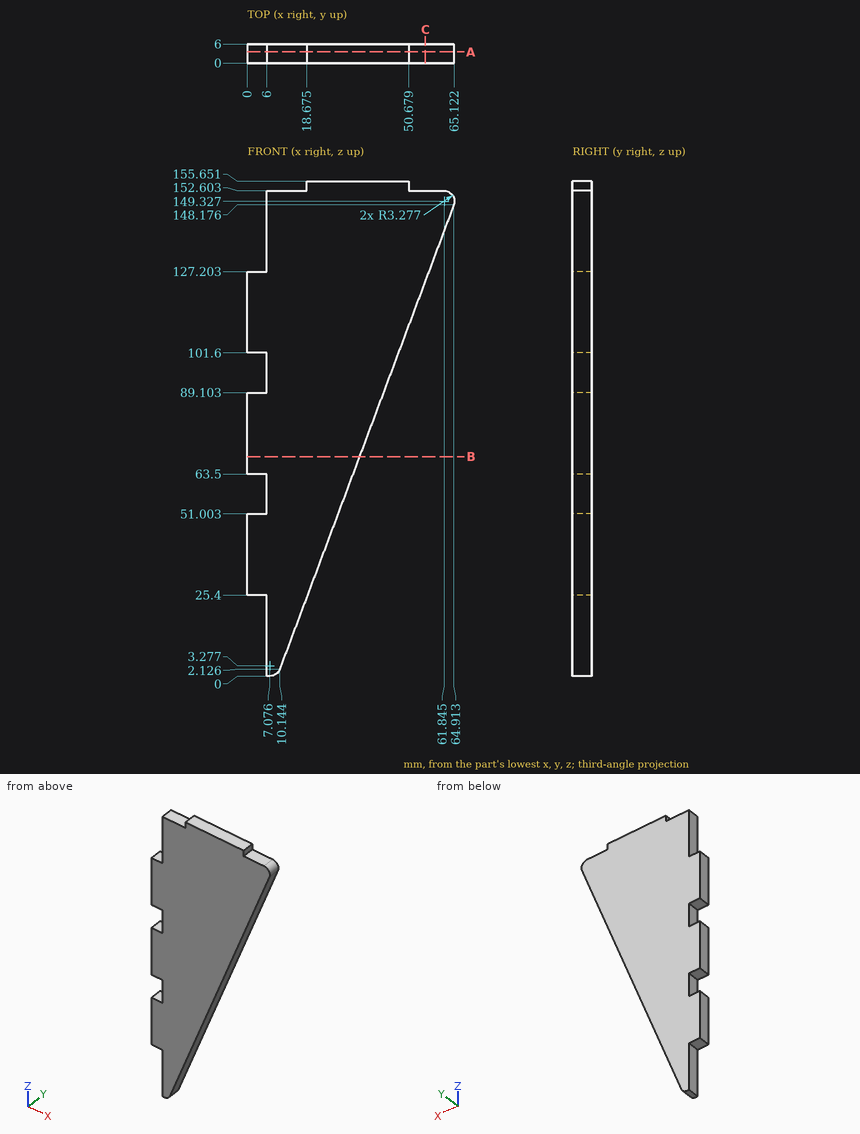
Design review of the part shown in the three views and the two pictorial views. Dimensions are in mm from the part's minimum x, y and z. Round coordinates to 2 decimals unless told otherwise and drop trailing zeros. Order: outer loops, then holes, each group sorted by start corner. A loop starts at its lowest first (then second) coordinate and runs counter-clockwise, first axis right, second up. Notation, with made-up numbers: (64, -7) - (115, -7) arc R23 ccw to (115, 22) - close; hole circle Ø8 at (85.25, -38). An arc over 180 degrees is marked (long way). One line per question, with ' | ' between items.
Item 1: For P1, Ø1.8, axis at x = 3, y = 4.5, coming from the -Z side; P2, Ø1.8, axis at y = 4, z = 58, coming from the -X side; P3, Ø3, axis at x = 2.5, y = 2, coming from the +Z side; P4, Ø3, axis at x = 33, z = 86.5, coming from the -Y side, all flat-tipped, find the tip position at first contact; note any pin that passes through.
Checks:
P1: z = 25.4 | P2: x = 6 | P3: z = 127.2 | P4: y = 0
Item 2: Take a section at C-C, the plane x = 56. Write out the cut boundary in (y, z).
Checks:
outline: (0, 124.41) - (6, 124.41) - (6, 152.6) - (0, 152.6) - close
Item 3: Wall thickness on line 1 (Z direction, x = 4, y = 1.4); line 2 (X direction, y = 5.6, z = 144.5) (1 decimal); line 3 (X direction, y = 1.25, z = 119): over which ranges is each line inside the solid? List them lowest first. Write a range as [from, to].
Checks:
line 1: [25.4, 51], [63.5, 89.1], [101.6, 127.2] | line 2: [6, 63.5] | line 3: [0, 53.97]
Item 4: Take a section at A-A, the plane y = 3.5. Write out the cut boundary in (x, z) (1 decimal).
Checks:
outline: (0, 25.4) - (6, 25.4) - (6, 0) - (7.1, 0) arc R3.3 ccw to (10.1, 2.1) - (64.9, 148.2) arc R3.3 ccw to (61.8, 152.6) - (50.7, 152.6) - (50.7, 155.7) - (18.7, 155.7) - (18.7, 152.6) - (6, 152.6) - (6, 127.2) - (0, 127.2) - (0, 101.6) - (6, 101.6) - (6, 89.1) - (0, 89.1) - (0, 63.5) - (6, 63.5) - (6, 51) - (0, 51) - close
Item 5: Take a section at B-B, the plane z = 69. Write out the cut boundary in (x, y).
Checks:
outline: (0, 0) - (35.22, 0) - (35.22, 6) - (0, 6) - close
